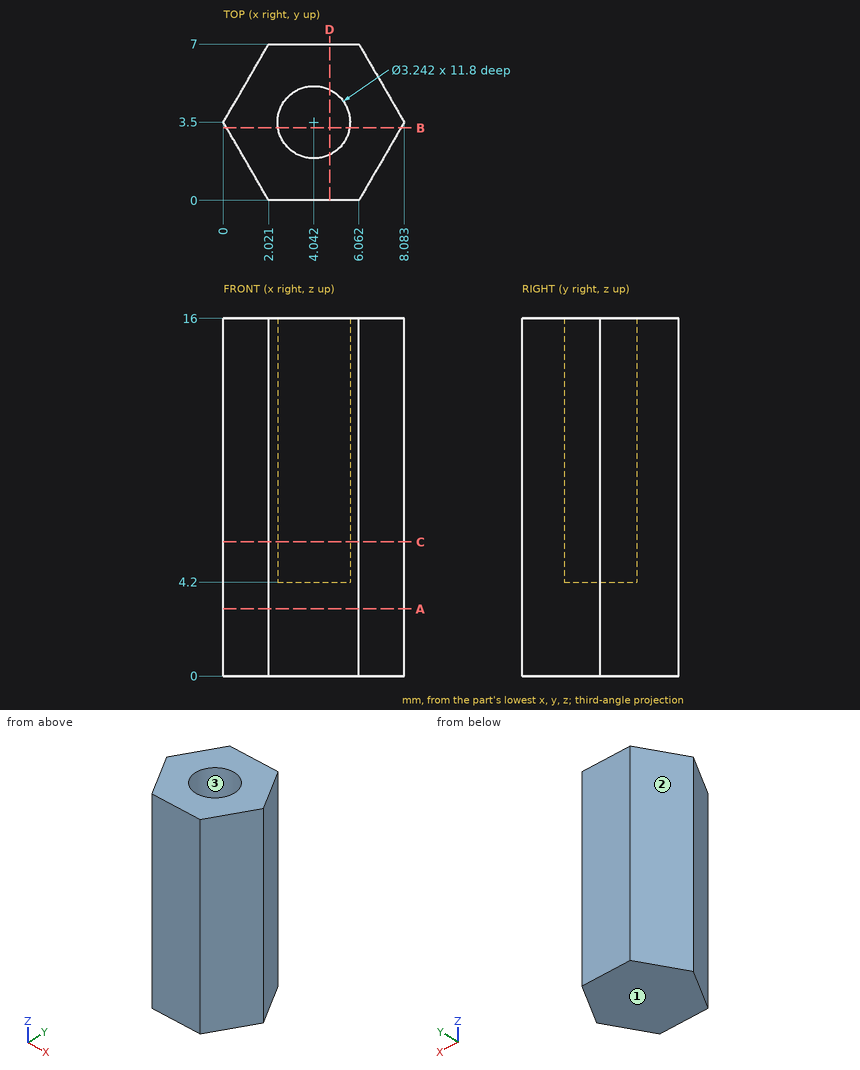
The figure shows three views and two pictorial views of one solid part (mm, origin at its lowest corner). Answer the questions. Give positions to 0.01 mm unless a question says otherwise; leave off trailing zeros. Order: outer loops, then holes, each group sorted by start corner. A loop starts at its lowest first (then second) coordinate and runs counter-clockwise, first axis right, second up. Notation, with made-up numbers: (79.25, 42.25) -> (115.25, 42.25) arc R6 ccw to (115.25, 51.25) -> close; hole circle Ø11 at (53.25, -21). An arc over 180 degrees is marked (long way). One line per item, written item: value.
1) Find section B-B, the plane y = 3.25. Determine the outline of the cut face in (x, z) (1 decimal).
Reported:
outline: (0.1, 0) -> (7.9, 0) -> (7.9, 16) -> (5.6, 16) -> (5.6, 4.2) -> (2.4, 4.2) -> (2.4, 16) -> (0.1, 16) -> close
2) Find section A-A, the plane z = 3. Determine the outline of the cut face in (x, y).
Reported:
outline: (0, 3.5) -> (2.02, 0) -> (6.06, 0) -> (8.08, 3.5) -> (6.06, 7) -> (2.02, 7) -> close
3) Determine the mould class of the marked faces 1, 2 and 3 for opening direction Y: pulls with the +Y half, pulls with the -Y half, needs draft (parallel to the pull), parting line crosses it, or undercut.
Reported:
face 1: needs draft
face 2: pulls with the +Y half
face 3: undercut
4) Flat-ended cylindrical pins translate along their axes: P1, Ø4, axis at y = 3.5, z = 8, coming from the -X side; P2, Ø1, axis at y = 6, z = 7, coming from the +X side; P3, Ø1.5, axis at x = 1, z = 8.5, coming from the -Y side. Find the tip coordinate at first contact, or state that the pin passes through.
Reported:
P1: stops at x = 0
P2: stops at x = 6.93
P3: stops at y = 0.47
5) Find section C-C, the plane z = 6. Determine the outline of the cut face in (x, y).
Reported:
outline: (0, 3.5) -> (2.02, 0) -> (6.06, 0) -> (8.08, 3.5) -> (6.06, 7) -> (2.02, 7) -> close; hole circle Ø3.24 at (4.04, 3.5)
6) Find section D-D, the plane x = 4.75. Determine the outline of the cut face in (y, z).
Reported:
outline: (0, 0) -> (7, 0) -> (7, 16) -> (4.96, 16) -> (4.96, 4.2) -> (2.04, 4.2) -> (2.04, 16) -> (0, 16) -> close
7) Find the intervals of material crossed by line 1 (X direction, y = 3.25, z = 13) (1 decimal); line 2 (Y direction, x = 3.25, z = 10.75) (1 decimal); line 3 (Z direction, x = 3, y = 3.5), in increasing order.
Reported:
line 1: x = 0.1 to 2.4, 5.6 to 7.9
line 2: y = 0 to 2.1, 4.9 to 7
line 3: z = 0 to 4.2
